For this review, take the finished solid that the model builds, in its own axes (mm). Coordinates: 2 decimals unless noted, no trailing zeros.
```python
from build123d import *

# Parameters (mm, degrees)
SKETCH1_W                    = 1212.85
SKETCH1_H                    = 316.23
BOSS_EXTRUDE1_DEPTH          = 3.175
FILLET1_R                    = 3.175
SKETCH4_W                    = 215.9
SKETCH4_H                    = 120.65
CUT_EXTRUDE1_DEPTH           = 1254.402016922
FILLET2_R                    = 3.175
F_10_0_1935_DIAMETER_HOLE1_D = 4.9149
F_1_4_0_25_DIAMETER_HOLE1_D  = 6.35


with BuildPart() as part:
    # Sketch1 → Boss-Extrude1 (new body)
    with BuildSketch(Plane(origin=(0, 0, 0), x_dir=(1, 0, 0), z_dir=(0, 1, 0))):
        with Locations((606.425, 158.115)):
            Rectangle(SKETCH1_W, SKETCH1_H)
    extrude(amount=BOSS_EXTRUDE1_DEPTH)

    # Fillet1
    fillet1_edges = [part.edges().sort_by_distance(p)[0] for p in [
        (606.425, 0, 0),
    ]]
    fillet(fillet1_edges, radius=FILLET1_R - 0.0001)  # a hair under: the kernel refuses the full size

    # Sketch4 → Cut-Extrude1 (cut, through all)
    with BuildSketch(Plane(origin=(0, 3.175, 0), x_dir=(1, 0, 0), z_dir=(0, 1, 0))):
        with Locations((301.625, 255.905)):
            Rectangle(SKETCH4_W, SKETCH4_H)
        with Locations((911.225, 255.905)):
            Rectangle(SKETCH4_W, SKETCH4_H)
    extrude(amount=-CUT_EXTRUDE1_DEPTH, mode=Mode.SUBTRACT)

    # Fillet2
    fillet2_edges = [part.edges().sort_by_distance(p)[0] for p in [
        (193.675, 1.5875, -195.58),
        (193.675, 1.5875, -316.23),
        (409.575, 1.5875, -316.23),
        (409.575, 1.5875, -195.58),
        (803.275, 1.5875, -316.23),
        (1019.175, 1.5875, -316.23),
        (1019.175, 1.5875, -195.58),
        (803.275, 1.5875, -195.58),
        (0, 1.5875, -316.23),
        (1212.85, 1.5875, -316.23),
    ]]
    fillet(fillet2_edges, radius=FILLET2_R)

    # #10 (0.1935) Diameter Hole1 (through all)
    with Locations(Plane(origin=(0, 3.175, 0), x_dir=(1, 0, 0), z_dir=(0, 1, 0))):
        with Locations((12.7, 193.675), (12.7, 247.65), (12.7, 288.925), (593.725, 193.675), (593.725, 247.65), (593.725, 288.925), (619.125, 288.925), (619.125, 247.65), (619.125, 193.675), (1200.15, 288.925), (1200.15, 247.65), (1200.15, 193.675)):
            Hole(F_10_0_1935_DIAMETER_HOLE1_D / 2)

    # 1/4 (0.25) Diameter Hole1 (through all)
    with Locations(Plane(origin=(0, 3.175, 0), x_dir=(1, 0, 0), z_dir=(0, 1, 0))):
        with Locations((193.675, 155.575), (193.675, 117.475), (428.625, 155.575), (428.625, 117.475), (784.225, 117.475), (784.225, 155.575), (1019.175, 117.475), (1019.175, 155.575)):
            Hole(F_1_4_0_25_DIAMETER_HOLE1_D / 2)


solid = part.part
```
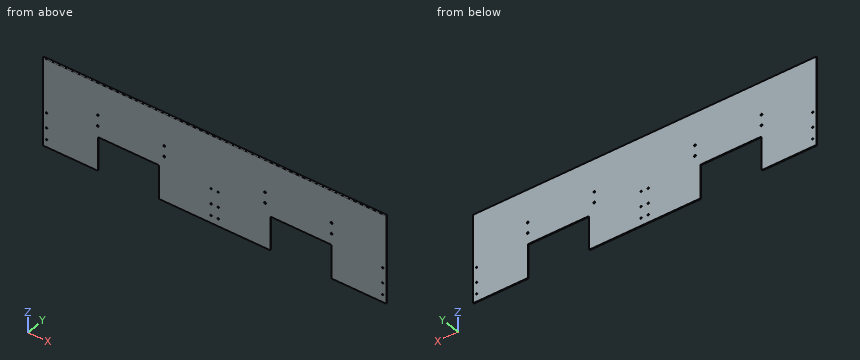
Q1. Clearance check with flat-ended pins moving along their axes: pin 1 Ø8 at (x, z) = (593.725, -193.675) entering from -Y; pin 2 Ø1.6 at (x, y) = (253, 1) entering from -Z. State where each tip first meets the part, or that it passes through.
Ans:
pin 1: stops at y = 0
pin 2: stops at z = -195.58
Q2. Add section B-B (y = 2.35). Give the number of separate pieces and of enclosed holes in the cut face, then the cut area to 3 significant figures.
Ans:
separate pieces: 1
enclosed holes: 20
area: 331,000 mm2
Q3. For probe 1 along X at (y, z) = (0.35, -230.5) (3 decimals); probe 2 along X at (y, z) = (1.7, -156); probe 3 along Z at (x, y) = (12.7, 0.85), list the stretches that pass through material, from the lowest coordinate up.
Ans:
probe 1: x = 0 to 193.675, 409.575 to 803.275, 1019.175 to 1212.85
probe 2: x = 0 to 190.53, 196.82 to 425.48, 431.77 to 781.08, 787.37 to 1016.03, 1022.32 to 1212.85
probe 3: z = -316.23 to -291.38, -286.47 to -250.11, -245.19 to -196.13, -191.22 to -1.01
